Geometry check sheet. Reference: the model listing, model coordinates, mm. A direction names the side the tool comes from. Round coordinates to 2 decimals unless told otherwise and drop trailing zeros. Write each loop counter-clockwise with the first axis right and the second up, starting at its lowest first coordinate (ties: lowest second). Pieces come first, ordered by that corner, then holes. Notation, with made-up numbers: (84.25, -31.75) -> (95.25, -31.75) arc R28 cw to (95.25, -12.75) -> close; hole circle Ø8 at (15.25, 59). An arc over 180 degrees is marked (long way). One line per question, with ' | ' between items.
Autodesk Inventor part; units mm, degrees
ref_plane "YZ Plane" through (0, 0, 0) normal (1, 0, 0) x (0, 1, 0)
ref_plane "XZ Plane" through (0, 0, 0) normal (0, 1, 0) x (-1, 0, 0)
ref_plane "XY Plane" through (0, 0, 0) normal (0, 0, 1) x (1, 0, 0)
sketch "Sketch1" plane through (0, 0, 0) normal (1, 0, 0) x (0, 1, 0)
  circle A0 centre (0, 0) radius 3.75
  circle A1 centre (0, 0) radius 6
  circle A2 centre (0, 0) radius 1.8
  dimension "d0" = 7.5
  dimension "d1" = 12
  dimension "d2" = 3.6
extrude "Extrusion1" add sketch "Sketch1" along normal blind 100 contours A0 | A1 | A2
extrude "Extrusion3" add sketch "Sketch1" against normal blind 2 contours A0
sketch "Sketch2" plane through (100, 0, 0) normal (1, 0, 0) x (0, 0, -1)
  circle A0 centre (0, 0) radius 3.75
  dimension "d9" = 7.5
extrude "Extrusion4" add sketch "Sketch2" along normal blind 2
extrude "Extrusion2" cut sketch "Sketch1" along normal blind 600 contours A2
properties part number "extendo100"
(1) Draft check along Y on faces 1 (the cylindrical face through (49, -6, 0)), 2 (the flat face through (0, -3, -3)), 3 (the cylindrical face through (50.728, 1.717, 0.541)). Enter one of: +Y half, -Y half, draft (parallel to the pull), parting line (faces both ways), or undercut.
Resolved:
face 1: parting line | face 2: draft | face 3: undercut
(2) Sectioned sample at A-A on y = 0. Record the cut outline in (x, z), then the cut area to 3 significant figures.
Resolved:
outline: (-2, -3.75) -> (0, -3.75) -> (0, -6) -> (100, -6) -> (100, -3.75) -> (102, -3.75) -> (102, -1.8) -> (-2, -1.8) -> close; (-2, 1.8) -> (102, 1.8) -> (102, 3.75) -> (100, 3.75) -> (100, 6) -> (0, 6) -> (0, 3.75) -> (-2, 3.75) -> close | area: 856 mm2
(3) Material ranges on line 1 (Z direction, x = 88.5, y = 0); line 2 (X direction, y = -4.25, z = 1); line 3 (Z direction, x = 38.5, y = 0.75), recorded low to high.
Resolved:
line 1: z = -6 to -1.8, 1.8 to 6 | line 2: x = 0 to 100 | line 3: z = -5.95 to -1.64, 1.64 to 5.95
(4) Access from +Z, -Z, +X, -X, +Y, -Y to the whole of each face (thin tool, end or side, straight path). Record for faces 4 (the cylindrical face through (100.986, -0.165, 3.746)), 5 (the flat face through (-2, 2, 1)), 6 (the cylindrical face through (-0.986, -3.746, 0.165)).
Resolved:
face 4: +X | face 5: +Z, -Z, -X, +Y, -Y | face 6: -X
(5) Sectioned sample at C-C on x = 34.5. Record the cut outline in (y, z), then the cut area to 3 significant figures.
Resolved:
outline: circle Ø12 at (0, 0); hole circle Ø3.6 at (0, 0) | area: 103 mm2
(6) Go/stop test with flat-tipped pins: pin 1 (3 mm diameter, centred on x = 42, y = -4, fed in from +Z); pin 2 (5 mm diameter, centred on x = 90, z = -3.5, fed in from +Y); pin 3 (3 mm diameter, centred on x = 69, z = 3.5, fed in from -Y). Record where each tip stops, or that it passes through.
Resolved:
pin 1: stops at z = 5.45 | pin 2: stops at y = 5.92 | pin 3: stops at y = -5.66
